Check sheet for the modelled part. Datum: model origin and axes. Units: mm. A direction names the side the tool comes from. Coordinates: 2 decimals unless noted, no trailing zeros. Write each loop counter-clockwise with the first axis right and the second up, starting at its lowest first coordinate (ties: lowest second). Pieces come first, ordered by that corner, then holes. Notation, with made-up numbers: M 69,4 L 122,4 A27 cw 122,36 Z; hole C 17,-14 d7. An arc over 180 degrees is marked long. Answer as CSV lines item,"result".
from build123d import *

# Parameters (mm, degrees)
F0_R     = 0.254
F1_DEPTH = 0.7874
F3_R     = 0.254
F4_DEPTH = 0.7874
F6_DEPTH = 20.828


with BuildPart() as f1:
    # F0 (on Front) → F1 (new body)
    with BuildSketch(Plane.XZ):
        with BuildLine():
            ThreePointArc((11.6844989808, 0.4963730507), (5.8365327764, 0.3827565605), (0, 0))
            Line((0, 0), (0, -5.5626))
            ThreePointArc((0, -5.5626), (0.2306241205, -6.1193758795), (0.7874, -6.35))
            ThreePointArc((0.7874, -6.35), (12.0142, -5.8528021894), (23.241, -6.35))
            ThreePointArc((23.241, -6.35), (23.7977758795, -6.1193758795), (24.0284, -5.5626))
            Line((24.0284, -5.5626), (24.0284, -3.1242))
            ThreePointArc((24.0284, -3.1242), (24.2032416576, -2.6294565946), (24.6501196779, -2.3544280917))
            ThreePointArc((24.6501196779, -2.3544280917), (24.7324922592, -2.3412194253), (24.8158, -2.3368))
            ThreePointArc((24.8158, -2.3368), (27.1526, -2.2171018645), (29.4894, -2.3368))
            ThreePointArc((29.4894, -2.3368), (29.7588076836, -2.2252076836), (29.8704, -1.9558))
            Line((29.8704, -1.9558), (29.8704, -0.9410763709))
            ThreePointArc((29.8704, -0.9410763709), (29.7800115236, -0.6946906116), (29.551733636, -0.5652100145))
            ThreePointArc((29.551733636, -0.5652100145), (29.5361211708, -0.563277779), (29.5205083425, -0.5613484801))
            ThreePointArc((29.5205083425, -0.5613484801), (26.1001935921, -0.2102344907), (22.6683376095, 0))
            ThreePointArc((22.6683376095, 0), (22.6321939395, -0.0149711983), (22.6172227412, -0.0511148683))
            Line((22.6172227412, -0.0511148683), (22.6172227412, -0.0581227141))
            ThreePointArc((22.6172227412, -0.0581227141), (22.602251543, -0.0942663841), (22.566107873, -0.1092375824))
            Line((22.566107873, -0.1092375824), (17.9650057107, -0.1092375824))
            Line((17.9650057107, -0.1092375824), (12.0393844661, 0.3669160007))
            ThreePointArc((12.0393844661, 0.3669160007), (12.0059153191, 0.3832006761), (11.9923637391, 0.4178666411))
            Line((11.9923637391, 0.4178666411), (11.9923637391, 0.4310297886))
            ThreePointArc((11.9923637391, 0.4310297886), (11.9792742883, 0.4651882045), (11.9467098063, 0.481852106))
            ThreePointArc((11.9467098063, 0.481852106), (11.8157921856, 0.4925036183), (11.6844989808, 0.4963730507))
        make_face()
        with Locations((1.778, -4.4702755668)):
            Circle(F0_R, mode=Mode.SUBTRACT)
        with Locations((4.0603091472, -4.2884453677)):
            Circle(F0_R, mode=Mode.SUBTRACT)
        with Locations((6.3296015834, -4.1486253579)):
            Circle(F0_R, mode=Mode.SUBTRACT)
    extrude(amount=F1_DEPTH)



with BuildPart() as f4:
    # F3 (on offset) → F4 (new body)
    with BuildSketch(Plane.XZ.offset(20.5994)):
        with BuildLine():
            ThreePointArc((11.6844989808, 0.4963730507), (5.8365327764, 0.3827565605), (0, 0))
            Line((0, 0), (0, -5.5626))
            ThreePointArc((0, -5.5626), (0.2306241205, -6.1193758795), (0.7874, -6.35))
            ThreePointArc((0.7874, -6.35), (12.0142, -5.8528021894), (23.241, -6.35))
            ThreePointArc((23.241, -6.35), (23.7977758795, -6.1193758795), (24.0284, -5.5626))
            Line((24.0284, -5.5626), (24.0284, -3.1242))
            ThreePointArc((24.0284, -3.1242), (24.2032416576, -2.6294565946), (24.6501196779, -2.3544280917))
            ThreePointArc((24.6501196779, -2.3544280917), (24.7324922592, -2.3412194253), (24.8158, -2.3368))
            ThreePointArc((24.8158, -2.3368), (27.1526, -2.2171018645), (29.4894, -2.3368))
            ThreePointArc((29.4894, -2.3368), (29.7588076836, -2.2252076836), (29.8704, -1.9558))
            Line((29.8704, -1.9558), (29.8704, -0.9410763709))
            ThreePointArc((29.8704, -0.9410763709), (29.7800115236, -0.6946906116), (29.551733636, -0.5652100145))
            ThreePointArc((29.551733636, -0.5652100145), (29.5361211708, -0.563277779), (29.5205083425, -0.5613484801))
            ThreePointArc((29.5205083425, -0.5613484801), (26.1001935921, -0.2102344907), (22.6683376095, 0))
            ThreePointArc((22.6683376095, 0), (22.6321939395, -0.0149711983), (22.6172227412, -0.0511148683))
            Line((22.6172227412, -0.0511148683), (22.6172227412, -0.0581227141))
            ThreePointArc((22.6172227412, -0.0581227141), (22.602251543, -0.0942663841), (22.566107873, -0.1092375824))
            Line((22.566107873, -0.1092375824), (17.9650057107, -0.1092375824))
            Line((17.9650057107, -0.1092375824), (12.0393844661, 0.3669160007))
            ThreePointArc((12.0393844661, 0.3669160007), (12.0059153191, 0.3832006761), (11.9923637391, 0.4178666411))
            Line((11.9923637391, 0.4178666411), (11.9923637391, 0.4310297886))
            ThreePointArc((11.9923637391, 0.4310297886), (11.9792742883, 0.4651882045), (11.9467098063, 0.481852106))
            ThreePointArc((11.9467098063, 0.481852106), (11.8157921856, 0.4925036183), (11.6844989808, 0.4963730507))
        make_face()
        with Locations((1.778, -4.4702755668)):
            Circle(F3_R, mode=Mode.SUBTRACT)
        with Locations((4.0603091472, -4.2884453677)):
            Circle(F3_R, mode=Mode.SUBTRACT)
        with Locations((6.3296015834, -4.1486253579)):
            Circle(F3_R, mode=Mode.SUBTRACT)
        with BuildLine():
            ThreePointArc((24.8158, -2.3368), (24.7324922592, -2.3412194253), (24.6501196779, -2.3544280917))
            ThreePointArc((24.6501196779, -2.3544280917), (24.7329437855, -2.345463165), (24.8158, -2.3368))
        make_face()
        with BuildLine():
            ThreePointArc((29.5205083425, -0.5613484801), (29.5361211708, -0.563277779), (29.551733636, -0.5652100145))
            ThreePointArc((29.551733636, -0.5652100145), (29.5361608672, -0.5629567849), (29.5205083425, -0.5613484801))
        make_face()
    extrude(amount=F4_DEPTH)


with BuildPart() as f1_1:
    add(f1.part)

    add(f4.part)  # F6 merges F4
    # F5 (on face) → F6 (join)
    with BuildSketch(Plane.XZ.offset(21.3868)):
        with BuildLine():
            ThreePointArc((29.551733636, -1.3526100145), (29.7800115236, -1.4820906116), (29.8704, -1.7284763709))
            Line((29.8704, -1.7284763709), (29.8704, -0.9410763709))
            ThreePointArc((29.8704, -0.9410763709), (29.7800115236, -0.6946906116), (29.551733636, -0.5652100145))
            ThreePointArc((29.551733636, -0.5652100145), (29.5361211708, -0.563277779), (29.5205083425, -0.5613484801))
            ThreePointArc((29.5205083425, -0.5613484801), (26.1001935921, -0.2102344907), (22.6683376095, 0))
            ThreePointArc((22.6683376095, 0), (22.6321939395, -0.0149711983), (22.6172227412, -0.0511148683))
            Line((22.6172227412, -0.0511148683), (22.6172227412, -0.0581227141))
            ThreePointArc((22.6172227412, -0.0581227141), (22.602251543, -0.0942663841), (22.566107873, -0.1092375824))
            Line((22.566107873, -0.1092375824), (17.9650057107, -0.1092375824))
            Line((17.9650057107, -0.1092375824), (12.0393844661, 0.3669160007))
            ThreePointArc((12.0393844661, 0.3669160007), (12.0059153191, 0.3832006761), (11.9923637391, 0.4178666411))
            Line((11.9923637391, 0.4178666411), (11.9923637391, 0.4310297886))
            ThreePointArc((11.9923637391, 0.4310297886), (11.9792742883, 0.4651882045), (11.9467098063, 0.481852106))
            ThreePointArc((11.9467098063, 0.481852106), (11.8157921856, 0.4925036183), (11.6844989808, 0.4963730507))
            ThreePointArc((11.6844989808, 0.4963730507), (5.8365327764, 0.3827565605), (0, 0))
            Line((0, 0), (0, -0.7874))
            ThreePointArc((0, -0.7874), (5.8365327764, -0.4046434395), (11.6844989808, -0.2910269493))
            ThreePointArc((11.6844989808, -0.2910269493), (11.8157921856, -0.2948963817), (11.9467098063, -0.305547894))
            ThreePointArc((11.9467098063, -0.305547894), (11.9792742883, -0.3222117955), (11.9923637391, -0.3563702114))
            Line((11.9923637391, -0.3563702114), (11.9923637391, -0.3695333589))
            ThreePointArc((11.9923637391, -0.3695333589), (12.0059153191, -0.4041993239), (12.0393844661, -0.4204839993))
            Line((12.0393844661, -0.4204839993), (17.9650057107, -0.8966375824))
            Line((17.9650057107, -0.8966375824), (22.566107873, -0.8966375824))
            ThreePointArc((22.566107873, -0.8966375824), (22.602251543, -0.8816663841), (22.6172227412, -0.8455227141))
            Line((22.6172227412, -0.8455227141), (22.6172227412, -0.8385148683))
            ThreePointArc((22.6172227412, -0.8385148683), (22.6321939395, -0.8023711983), (22.6683376095, -0.7874))
            ThreePointArc((22.6683376095, -0.7874), (26.1001935921, -0.9976344907), (29.5205083425, -1.3487484801))
            ThreePointArc((29.5205083425, -1.3487484801), (29.5361608672, -1.3503567849), (29.551733636, -1.3526100145))
        make_face()
    extrude(amount=-F6_DEPTH)


solid = f1_1.part
1) Mould release check, pull along Y, two halves, no side actions. Record for faces 1 (the face through (26.052, -10.832, -0.994)), 2 (the face through (11, 0, -3)), 3 (the face through (26.148, -10.544, -0.214)): pulls with the +Y half, pulls with the -Y half, needs draft (parallel to the pull), parting line crosses it, or undercut.
Answer key:
face 1,"undercut"
face 2,"pulls with the +Y half"
face 3,"needs draft"
2) Section check A-A, the plane z = -3.5. Record the boundary of the cut face in (x, y), plus the area to 3 significant figures.
Answer key:
outline,"M 0,-21.39 L 24.03,-21.39 L 24.03,-20.6 L 0,-20.6 Z; M 0,-0.79 L 24.03,-0.79 L 24.03,0 L 0,0 Z"
area,"37.8 mm2"
3) Depth check by flat-ended pin: P1, Ø3, axis at x = 22.5, y = -17, coming from the -Z side; P2, Ø0.9, axis at y = -0.5, z = -4, coming from the +X side; P3, Ø1.4, axis at x = 20, y = -12.5, coming from the +Z side. Enter the tip coordinate at first touch or a pass-through.
Answer key:
P1,"stops at z = -0.9"
P2,"stops at x = 24.03"
P3,"stops at z = -0.11"
4) Section check C-C, the plane x = 17.5. Record the boundary of the cut face in (y, z), plus the area to 3 significant figures.
Answer key:
outline,"M -21.39,-5.97 L -20.6,-5.97 L -20.6,-0.86 L -0.79,-0.86 L -0.79,-5.97 L 0,-5.97 L 0,-0.07 L -21.39,-0.07 Z"
area,"24.9 mm2"
5) Thickness scan on line 1 along Y through (x, z) = (7.75, -4.75); line 2 along Z through (x, y) = (17.25, -4.25); line 3 along Z through (x, y) = (9, -18.5). Record the ranges inside material, lowest first.
Answer key:
line 1,"y = -21.39 to -20.6, -0.79 to 0"
line 2,"z = -0.84 to -0.05"
line 3,"z = -0.31 to 0.48"
6) Tool access check on faces 4 (the face through (20, -11, -0.897)), 5 (the face through (5.75, -10.83, -0.41)), 6 (the face through (11, -21.387, -3)), 7 (the face through (15.044, -10.544, 0.126)). Record the directions out of +Z, -Z, +X, -X, +Y, -Y that give a thin tool (end or side, any length) a straight path to the whole face; none if there is none.
Answer key:
face 4,"-Z, -X"
face 5,"-Z"
face 6,"+Z, -Z, +X, -X, -Y"
face 7,"+Z, +Y, -Y"
7) Section check D-D, the plane x = 22. Record the boundary of the cut face in (y, z).
Answer key:
outline,"M -21.39,-6.25 L -20.6,-6.25 L -20.6,-0.9 L -0.79,-0.9 L -0.79,-6.25 L 0,-6.25 L 0,-0.11 L -21.39,-0.11 Z"
